from build123d import *

# Parameters (mm, degrees)
F0_R     = 2.75
F0_W     = 10
F0_H     = 5.1
F1_DEPTH = 70
F2_DEPTH = 45


# Not quite as in the source:
# - a feature names something its author has since deleted; it is built from what else it names


with BuildPart() as f1:
    # F0 (on Top) → F1 (new body)
    with BuildSketch(Plane.XY):
        with BuildLine():
            Line((-60, -60), (60, -60))
            Line((60, -60), (60, 60))
            Line((60, 60), (-60, 60))
            Line((-60, 60), (-60, 13.55))
            Line((-60, 13.55), (-40.5, 13.55))
            Line((-40.5, 13.55), (-40.5, 18.65))
            Line((-40.5, 18.65), (-30.5, 18.65))
            Line((-30.5, 18.65), (-30.5, 20.5))
            Line((-30.5, 20.5), (-25.5, 20.5))
            ThreePointArc((-25.5, 20.5), (-21.9644660941, 21.9644660941), (-20.5, 25.5))
            Line((-20.5, 25.5), (-20.5, 30.5))
            Line((-20.5, 30.5), (20.5, 30.5))
            Line((20.5, 30.5), (20.5, 25.5))
            ThreePointArc((20.5, 25.5), (21.9644660941, 21.9644660941), (25.5, 20.5))
            Line((25.5, 20.5), (30.5, 20.5))
            Line((30.5, 20.5), (30.5, -20.5))
            Line((30.5, -20.5), (25.5, -20.5))
            ThreePointArc((25.5, -20.5), (21.9644660941, -21.9644660941), (20.5, -25.5))
            Line((20.5, -25.5), (20.5, -30.5))
            Line((20.5, -30.5), (-20.5, -30.5))
            Line((-20.5, -30.5), (-20.5, -25.5))
            ThreePointArc((-20.5, -25.5), (-21.9644660941, -21.9644660941), (-25.5, -20.5))
            Line((-25.5, -20.5), (-30.5, -20.5))
            Line((-30.5, -20.5), (-30.5, -18.65))
            Line((-30.5, -18.65), (-30.5, -13.55))
            Line((-30.5, -13.55), (-40.5, -13.55))
            Line((-40.5, -13.55), (-60, -13.55))
            Line((-60, -13.55), (-60, -18.65))
            Line((-60, -18.65), (-60, -60))
        make_face()
        with Locations((-46, -46)):
            Circle(F0_R, mode=Mode.SUBTRACT)
        with Locations((46, -46)):
            Circle(F0_R, mode=Mode.SUBTRACT)
        with Locations((-46, 46)):
            Circle(F0_R, mode=Mode.SUBTRACT)
        with Locations((46, 46)):
            Circle(F0_R, mode=Mode.SUBTRACT)
        Polygon((-60, 13.55), (-60, -13.55), (-40.5, -13.55), (-30.5, -13.55), (-30.5, 13.55), (-40.5, 13.55), align=None)
        with BuildLine():
            Line((-30.5, 13.55), (-30.5, -13.55))
            Line((-30.5, -13.55), (-30.5, -18.65))
            Line((-30.5, -18.65), (-30.5, -20.5))
            Line((-30.5, -20.5), (-25.5, -20.5))
            ThreePointArc((-25.5, -20.5), (-21.9644660941, -21.9644660941), (-20.5, -25.5))
            Line((-20.5, -25.5), (-20.5, -30.5))
            Line((-20.5, -30.5), (20.5, -30.5))
            Line((20.5, -30.5), (20.5, -25.5))
            ThreePointArc((20.5, -25.5), (21.9644660941, -21.9644660941), (25.5, -20.5))
            Line((25.5, -20.5), (30.5, -20.5))
            Line((30.5, -20.5), (30.5, 20.5))
            Line((30.5, 20.5), (25.5, 20.5))
            ThreePointArc((25.5, 20.5), (21.9644660941, 21.9644660941), (20.5, 25.5))
            Line((20.5, 25.5), (20.5, 30.5))
            Line((20.5, 30.5), (-20.5, 30.5))
            Line((-20.5, 30.5), (-20.5, 25.5))
            ThreePointArc((-20.5, 25.5), (-21.9644660941, 21.9644660941), (-25.5, 20.5))
            Line((-25.5, 20.5), (-30.5, 20.5))
            Line((-30.5, 20.5), (-30.5, 18.65))
            Line((-30.5, 18.65), (-30.5, 13.55))
        make_face()
        with Locations((-35.5, 16.1)):
            Rectangle(F0_W, F0_H)
    extrude(amount=-F1_DEPTH)

    # F0 (on Top) → F2 (cut)
    with BuildSketch(Plane.XY):
        Polygon((-60, 13.55), (-60, -13.55), (-40.5, -13.55), (-30.5, -13.55), (-30.5, 13.55), (-40.5, 13.55), align=None)
        with BuildLine():
            Line((-30.5, 13.55), (-30.5, -13.55))
            Line((-30.5, -13.55), (-30.5, -18.65))
            Line((-30.5, -18.65), (-30.5, -20.5))
            Line((-30.5, -20.5), (-25.5, -20.5))
            ThreePointArc((-25.5, -20.5), (-21.9644660941, -21.9644660941), (-20.5, -25.5))
            Line((-20.5, -25.5), (-20.5, -30.5))
            Line((-20.5, -30.5), (20.5, -30.5))
            Line((20.5, -30.5), (20.5, -25.5))
            ThreePointArc((20.5, -25.5), (21.9644660941, -21.9644660941), (25.5, -20.5))
            Line((25.5, -20.5), (30.5, -20.5))
            Line((30.5, -20.5), (30.5, 20.5))
            Line((30.5, 20.5), (25.5, 20.5))
            ThreePointArc((25.5, 20.5), (21.9644660941, 21.9644660941), (20.5, 25.5))
            Line((20.5, 25.5), (20.5, 30.5))
            Line((20.5, 30.5), (-20.5, 30.5))
            Line((-20.5, 30.5), (-20.5, 25.5))
            ThreePointArc((-20.5, 25.5), (-21.9644660941, 21.9644660941), (-25.5, 20.5))
            Line((-25.5, 20.5), (-30.5, 20.5))
            Line((-30.5, 20.5), (-30.5, 18.65))
            Line((-30.5, 18.65), (-30.5, 13.55))
        make_face()
        with Locations((-35.5, 16.1)):
            Rectangle(F0_W, F0_H)
    extrude(amount=-F2_DEPTH, mode=Mode.SUBTRACT)


solid = f1.part
Part model, mm, in its own coordinate system. A direction names the side the tool comes from. Coordinates: 2 decimals unless noted, no trailing zeros. Write each loop counter-clockwise with the first axis right and the second up, starting at its lowest first coordinate (ties: lowest second). Pieces come first, ordered by that corner, then holes. Notation, with made-up numbers: M 16,73.5 L 33,73.5 A38 cw 33,112.5 Z; hole C -33.75,-23 d11. An arc over 180 degrees is marked long. Return JSON: item names as keys, results as strings.
1. Saw through at D-D, the plane z = -6. Count the separate pieces of the cut face and the enclosed holes in it, then the cut area to 3 significant figures.
Determined:
{"separate pieces": "1", "enclosed holes": "4", "area": "10,100 mm²"}
2. Flat gauge pins, fed straight in: pin 1 Ø3.5 at (x, y) = (46, -46) entering from -Z; pin 2 Ø18.5 at (x, y) = (-14, -3.5) entering from +Z; pin 3 Ø12.5 at (y, z) = (1.5, -30) entering from -X. Where does each tip first touch, or does it go through?
Determined:
{"pin 1": "through", "pin 2": "z = -45", "pin 3": "x = 30.5"}
3. Saw through at C-C, the plane x = -34. Write the cut outline in (y, z).
Determined:
{"outline": "M -60,-70 L 60,-70 L 60,0 L 18.65,0 L 18.65,-45 L -13.55,-45 L -13.55,0 L -60,0 Z"}
4. Probe L1, parallel to Y at x = 46, z = -14; L2, parallel to Y at x = -46, z = -40; L3, parallel to Y at x = -16, z = -37. List the from-to ranges inside material, lowest first.
Determined:
{"L1": "-60 to -48.75, -43.25 to 43.25, 48.75 to 60", "L2": "-60 to -48.75, -43.25 to -13.55, 13.55 to 43.25, 48.75 to 60", "L3": "-60 to -30.5, 30.5 to 60"}
5. 3-axis set-ups, long thin cutter, end or side, ignore diameter. For faces 4 (the face through (-30.5, -17, -22)), 5 (the face through (26, 28, 0)), 6 (the face through (-50, 13.55, -22)): which of +Z, -Z, +X, -X, +Y, -Y reach the whole face in a straight line?
Determined:
{"face 4": "+Z", "face 5": "+Z, +X, -X, +Y, -Y", "face 6": "+Z, -X"}
6. Saw through at A-A, the plane x = 46. Write the cut outline in (y, z).
Determined:
{"outline": "M -60,-70 L -48.75,-70 L -48.75,0 L -60,0 Z; M -43.25,-70 L 43.25,-70 L 43.25,0 L -43.25,0 Z; M 48.75,-70 L 60,-70 L 60,0 L 48.75,0 Z"}
7. Pull direction X, two halves, no side cores. Call faces 1 (the face through (-36, 18.65, -22)), 2 (the face through (28, 20.5, -22)), 3 (the face through (1, 60, -35)): pulls with the +X half, pulls with the -X half, needs draft (parallel to the pull), parting line crosses it, or undercut.
Determined:
{"face 1": "undercut", "face 2": "undercut", "face 3": "needs draft"}
